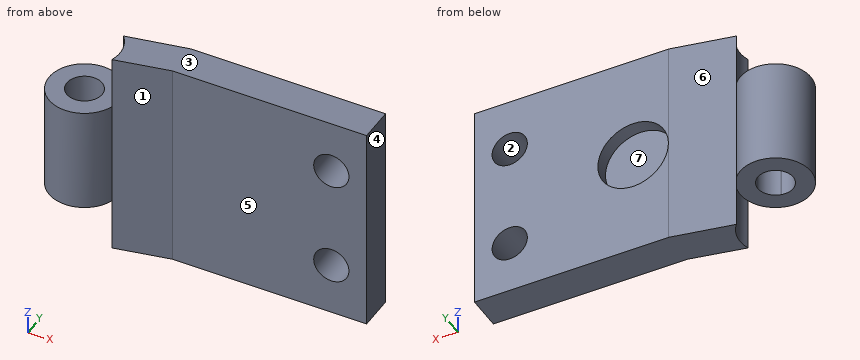
from build123d import *

# Parameters (mm, degrees)
Y_KSEKLIK_EKSTR_ZYON1_DEPTH = 30
KES_EKSTR_ZYON1_START       = -30
IZIM2_R                     = 2.5
KES_EKSTR_ZYON1_DEPTH       = 30
KES_EKSTR_ZYON3_START       = -7.5
IZIM6_R                     = 5
KES_EKSTR_ZYON3_DEPTH       = 7.5
IZIM7_R                     = 5
KES_EKSTR_ZYON4_DEPTH       = 7.5
IZIM9_R                     = 5
KES_EKSTR_ZYON6_DEPTH       = 2
IZIM10_R                    = 2.5
KES_EKSTR_ZYON7_DEPTH       = 5


with BuildPart() as part:
    # Çizim1 → Yükseklik-Ekstrüzyon1 (new body)
    with BuildSketch(Plane.XY):
        with BuildLine():
            Line((-25.050567114, 3.343092307), (-16.318399297, 5.056233526))
            Line((-16.318399297, 5.056233526), (3.922819568, 5.056233526))
            Line((3.922819568, 5.056233526), (6.182819568, 5.056233526))
            Line((6.182819568, 5.056233526), (11.182819568, 5.056233526))
            Line((11.182819568, 5.056233526), (11.182819568, 0.056233526))
            Line((11.182819568, 0.056233526), (6.182819568, 0.056233526))
            Line((6.182819568, 0.056233526), (3.922819568, 0.056233526))
            Line((3.922819568, 0.056233526), (-16.318399297, 0.056233526))
            Line((-16.318399297, 0.056233526), (-24.07574143, -1.527179355))
            ThreePointArc((-24.07574143, -1.527179355), (-33.721153292, -0.925093769), (-25.050567114, 3.343092307))
        make_face()
        with BuildLine():
            Line((-28.337105741, -2.397000362), (-28.299750993, -2.389375587))
            ThreePointArc((-28.299750993, -2.389375587), (-28.318413832, -2.393259183), (-28.337105741, -2.397000362))
        make_face(mode=Mode.SUBTRACT)
    extrude(amount=Y_KSEKLIK_EKSTR_ZYON1_DEPTH)

    # Çizim2 → Kes-Ekstrüzyon1 (cut)
    with BuildSketch(Plane.XY.offset(30).offset(KES_EKSTR_ZYON1_START)):
        with Locations((-28.818399297, 0.056233526)):
            Circle(IZIM2_R)
    extrude(amount=KES_EKSTR_ZYON1_DEPTH, mode=Mode.SUBTRACT)

    # Çizim6 → Kes-Ekstrüzyon3 (cut)
    with BuildSketch(Plane.XY.offset(30).offset(KES_EKSTR_ZYON3_START)):
        with Locations((-28.818399297, 0.056233526)):
            Circle(IZIM6_R)
    extrude(amount=KES_EKSTR_ZYON3_DEPTH, mode=Mode.SUBTRACT)

    # Çizim7 → Kes-Ekstrüzyon4 (cut)
    with BuildSketch(Plane(origin=(0, 0, 0), x_dir=(-1, 0, 0), z_dir=(0, 0, -1))):
        with Locations((28.818399297, 0.056233526)):
            Circle(IZIM7_R)
    extrude(amount=-KES_EKSTR_ZYON4_DEPTH, mode=Mode.SUBTRACT)

    # Çizim9 → Kes-Ekstrüzyon6 (cut)
    with BuildSketch(Plane(origin=(0, 5.056233526, 0), x_dir=(1, 0, 0), z_dir=(0, 1, 0))):
        with Locations(Location((-11.317180432, -15, 0), (0, 0, 270))):
            Circle(IZIM9_R)
    extrude(amount=-KES_EKSTR_ZYON6_DEPTH, mode=Mode.SUBTRACT)

    # Çizim10 → Kes-Ekstrüzyon7 (cut)
    with BuildSketch(Plane(origin=(0, 5.056233526, 0), x_dir=(1, 0, 0), z_dir=(0, 1, 0))):
        with Locations(Location((6.182819568, -22.5, 0), (0, 0, 270))):
            Circle(IZIM10_R)
        with Locations(Location((6.182819568, -7.5, 0), (0, 0, 270))):
            Circle(IZIM10_R)
    extrude(amount=-KES_EKSTR_ZYON7_DEPTH, mode=Mode.SUBTRACT)


solid = part.part
Build history of the part. All positions in model axes, mm. Face numbers are marked on the shaded views. A direction names the side the tool comes from. Coordinates: 2 decimals unless noted, no trailing zeros. Write each loop counter-clockwise with the first axis right and the second up, starting at its lowest first coordinate (ties: lowest second). Pieces come first, ordered by that corner, then holes. Notation, with made-up numbers: (69, -33) -> (80, -33) arc R34 cw to (80, 3) -> close; hole circle Ø11 at (29, 67.5). An arc over 180 degrees is marked (long way). Use CSV: the item, a comma, the result in double quotes. Start each with the question number.
Q1. Flat gauge pins, fed straight in: pin 1 Ø4 at (x, z) = (-20.5, 15.5) entering from +Y; pin 2 Ø5 at (x, z) = (-10.5, 14) entering from +Y; pin 3 Ø4 at (y, z) = (-2.5, 14) entering from -X. Where does each tip first touch, or does it go through?
Q2. Pull direction X, two halves, no side cores. Call the marked faces 1, 2 and 3: released by +X, released by -X, zero draft, split by the parting line, or undercut.
Q3. Cut at C-C, the plane x = -27.5. List the corners of the cut face in (y, z).
Q4. Cut at B-B, the plane y = 4.25. List the corners of the cut face in (x, z).
Q5. Cut at A-A, the plane z = 8. List the corners of the cut face in (x, y).
Q6. Drill centre lines: probe 1 along Z at (x, y) = (7.5, 2.25); probe 2 along X at (y, z) = (0.25, 7.75); probe 3 along Y at (x, z) = (-15, 10). Where is each one in solid material? Low to high.
Q7. 3-axis set-ups, long thin cutter, end or side, ignore diameter. For the marked faces 4, 5, 6 and 7: which of +Z, -Z, +X, -X, +Y, -Y reach the whole face in a straight line?
Checked values:
1,pin 1,"stops at y = 4.63"
1,pin 2,"stops at y = 3.06"
1,pin 3,"stops at x = -33.79"
2,face 1,"released by +X"
2,face 2,"undercut"
2,face 3,"zero draft"
3,outline,"(-4.77, 7.5) -> (-2.07, 7.5) -> (-2.07, 22.5) -> (-4.77, 22.5) -> close; (2.18, 7.5) -> (4.88, 7.5) -> (4.88, 22.5) -> (2.18, 22.5) -> close"
4,outline,"(-31.54, 7.5) -> (-26.1, 7.5) -> (-26.1, 22.5) -> (-31.54, 22.5) -> close; (-20.43, 0) -> (11.18, 0) -> (11.18, 30) -> (-20.43, 30) -> close; hole circle Ø10 at (-11.32, 15); hole circle Ø5 at (6.18, 7.5); hole circle Ø5 at (6.18, 22.5)"
5,outline,"(-25.05, 3.34) arc R5 ccw (long way) to (-24.08, -1.53) -> (-16.32, 0.06) -> (3.73, 0.06) -> (3.73, 5.06) -> (-16.32, 5.06) -> close; (8.63, 0.06) -> (11.18, 0.06) -> (11.18, 5.06) -> (8.63, 5.06) -> close; hole circle Ø5 at (-28.82, 0.06)"
6,probe 1,"z = 0 to 5.38, 9.62 to 20.38, 24.62 to 30"
6,probe 2,"x = -33.81 to -31.31, -26.33 to 3.7, 8.67 to 11.18"
6,probe 3,"y = 0.06 to 5.06"
7,face 4,"+Z, -Z, +X, +Y, -Y"
7,face 5,"+Z, -Z, +X, -Y"
7,face 6,"+Z, -Z, +Y"
7,face 7,"+Y"
